```python
from build123d import *

# Parameters (mm, degrees)
SKETCH1_W           = 22
SKETCH1_H           = 14
BOSS_EXTRUDE1_DEPTH = 10
SKETCH1_3_W         = 22
SKETCH1_3_H         = 14
BOSS_EXTRUDE2_DEPTH = 18
SKETCH1_4_W         = 22
SKETCH1_4_H         = 14
BOSS_EXTRUDE3_DEPTH = 32
CHAMFER1_SIZE       = 2
SKETCH2_R           = 3
CUT_EXTRUDE1_DEPTH  = 56.6596802


with BuildPart() as part:
    # Sketch1 → Boss-Extrude1 (new body)
    with BuildSketch(Plane(origin=(0, 0, 0), x_dir=(1, 0, 0), z_dir=(0, 1, 0))):
        with BuildLine():
            Line((0, 8), (0, 15))
            ThreePointArc((0, 15), (-15, 0), (0, -15))
            Line((0, -15), (0, -8))
            ThreePointArc((0, -8), (-8, 0), (0, 8))
        make_face()
        with BuildLine():
            Line((28, 7), (13.266499161, 7))
            ThreePointArc((13.266499161, 7), (7.745966692, 12.845232579), (0, 15))
            Line((0, 15), (0, 8))
            ThreePointArc((0, 8), (5.656854249, 5.656854249), (8, 0))
            ThreePointArc((8, 0), (5.656854249, -5.656854249), (0, -8))
            Line((0, -8), (0, -15))
            ThreePointArc((0, -15), (7.745966692, -12.845232579), (13.266499161, -7))
            Line((13.266499161, -7), (28, -7))
            Line((28, -7), (28, 7))
        make_face()
        with Locations((39, 0)):
            Rectangle(SKETCH1_W, SKETCH1_H)
    extrude(amount=BOSS_EXTRUDE1_DEPTH)

    # Sketch1_3 → Boss-Extrude2 (add)
    with BuildSketch(Plane(origin=(0, 0, 0), x_dir=(1, 0, 0), z_dir=(0, 1, 0))):
        with BuildLine():
            Line((28, 7), (13.266499161, 7))
            ThreePointArc((13.266499161, 7), (7.745966692, 12.845232579), (0, 15))
            Line((0, 15), (0, 8))
            ThreePointArc((0, 8), (5.656854249, 5.656854249), (8, 0))
            ThreePointArc((8, 0), (5.656854249, -5.656854249), (0, -8))
            Line((0, -8), (0, -15))
            ThreePointArc((0, -15), (7.745966692, -12.845232579), (13.266499161, -7))
            Line((13.266499161, -7), (28, -7))
            Line((28, -7), (28, 7))
        make_face()
        with Locations((39, 0)):
            Rectangle(SKETCH1_3_W, SKETCH1_3_H)
    extrude(amount=BOSS_EXTRUDE2_DEPTH)

    # Sketch1_4 → Boss-Extrude3 (add)
    with BuildSketch(Plane(origin=(0, 0, 0), x_dir=(1, 0, 0), z_dir=(0, 1, 0))):
        with Locations((39, 0)):
            Rectangle(SKETCH1_4_W, SKETCH1_4_H)
    extrude(amount=BOSS_EXTRUDE3_DEPTH)

    # Chamfer1
    chamfer1_edges = [part.edges().sort_by_distance(p)[0] for p in [
        (39, 32, -7),
        (39, 32, 7),
    ]]
    chamfer(chamfer1_edges, length=CHAMFER1_SIZE)

    # Sketch2 → Cut-Extrude1 (cut, through all)
    with BuildSketch(Plane.ZY.offset(-28)):
        with Locations((0, 24)):
            Circle(SKETCH2_R)
    extrude(amount=-CUT_EXTRUDE1_DEPTH, mode=Mode.SUBTRACT)


solid = part.part
```
Work out the finished part from the listing and answer in its coordinate system (mm). A direction names the side the tool comes from. Round coordinates to 2 decimals unless told otherwise and drop trailing zeros. Order: outer loops, then holes, each group sorted by start corner. A loop starts at its lowest first (then second) coordinate and runs counter-clockwise, first axis right, second up.
Q1. The mould has two halves that part along Y. Classify faces 1 (the cylindrical face through (38.85, 21.07, -0.65)), 2 (the flat face through (14, 18, 0)), 3 (the flat face through (35, 11, 7)): pulls with the +Y half, pulls with the -Y half, needs draft (parallel to the pull), parting line crosses it, or undercut.
Solution:
face 1: undercut
face 2: pulls with the +Y half
face 3: needs draft
Q2. A cutting plane is placed at C-C, the plane z = 0. Determine the outline of the cut face in (x, y).
Solution:
outline: (-15, 0) - (-8, 0) - (-8, 10) - (-15, 10) - close; (8, 0) - (50, 0) - (50, 21) - (28, 21) - (28, 18) - (8, 18) - close; (28, 27) - (50, 27) - (50, 32) - (28, 32) - close
Q3. A cutting plane is placed at B-B, the plane y = 3. Determine the outline of the cut face in (x, z), then the cut area to 3 significant figures.
Solution:
outline: (13.27, -7) - (50, -7) - (50, 7) - (13.27, 7) arc R15 ccw (long way) to start; hole circle Ø16 at (0, 0)
area: 1,000 mm2
Q4. A tool of negligible diameter and unlimited length cuts with its end or side. For faces 4 (the flat face through (-9, 10, 0)), 5 (the flat face through (36, 11, -7)), 6 (the flat face through (39, 31, 6)), from which of +Z, -Z, +X, -X, +Y, -Y can it reach the whole face along a straight path? Write none if from no direction.
Solution:
face 4: +Z, -Z, -X, +Y
face 5: -Z, +X, +Y, -Y
face 6: +Z, +X, -X, +Y
Q5. A cutting plane is placed at D-D, the plane x = 31. Determine the outline of the cut face in (y, z), then the cut area to 3 significant figures.
Solution:
outline: (0, -7) - (30, -7) - (32, -5) - (32, 5) - (30, 7) - (0, 7) - close; hole circle Ø6 at (24, 0)
area: 416 mm2
Q6. Given pin 1 Ø7 at (y, z) = (26, 1) entering from -X; pin 2 Ø3.5 at (y, z) = (15.5, -11.5) entering from -X; pin 3 Ø15 at (x, y) = (38.5, 20.5) entering from +Z; pin 4 Ø13 at (x, z) = (0, 0) entering from +Y, each flat-ended and moving along its own axis, determine where each tip first touches the part or whether it passes through.
Solution:
pin 1: stops at x = 28
pin 2: stops at x = 0
pin 3: stops at z = 7
pin 4: passes through
Q7. A cutting plane is placed at A-A, the plane y = 24. Determine the outline of the cut face in (x, z).
Solution:
outline: (28, -7) - (50, -7) - (50, -3) - (28, -3) - close; (28, 3) - (50, 3) - (50, 7) - (28, 7) - close
Q8. Find the intervals of material crossed by line 1 along Y through (x, z) = (36.25, 0); line 2 along X through (y, z) = (9, 0); line 3 along Y through (x, z) = (4, 14), in increasing order.
Solution:
line 1: y = 0 to 21, 27 to 32
line 2: x = -15 to -8, 8 to 50
line 3: y = 0 to 18
